Geometry check sheet. Reference: the model listing, model coordinates, mm. A direction names the side the tool comes from. Coordinates: 2 decimals unless noted, no trailing zeros. Order: outer loops, then holes, each group sorted by start corner. A loop starts at its lowest first (then second) coordinate and runs counter-clockwise, first axis right, second up. Notation, with made-up numbers: (0, 18) -> (10, 18) arc R12 cw to (10, 22) -> close; hole circle Ø4 at (-23, 11.25). An arc over 180 degrees is marked (long way). Answer in a Markdown table with one row per item. Add a question column.
```python
from build123d import *

# Parameters (mm, degrees)
F0_R     = 7.5
F1_DEPTH = 10
F2_DEPTH = 20
F3_R     = 2.5
F4_DEPTH = 3.9289322881


with BuildPart() as f1:
    # F0 (on Front) → F1 (new body)
    with BuildSketch(Plane.XZ):
        with BuildLine():
            Line((11.1803398875, 10), (-11.1803398875, 10))
            ThreePointArc((-11.1803398875, 10), (0, -15), (11.1803398875, 10))
        make_face()
        Circle(F0_R, mode=Mode.SUBTRACT)
        with BuildLine():
            ThreePointArc((11.1803398875, 10), (0, -15), (-11.1803398875, 10))
            Line((-11.1803398875, 10), (-20.1556443707, 10))
            ThreePointArc((-20.1556443707, 10), (0, -22.5), (20.1556443707, 10))
            Line((20.1556443707, 10), (11.1803398875, 10))
        make_face()
    extrude(amount=F1_DEPTH)

    # F0 (on Front) → F2 (join)
    with BuildSketch(Plane.XZ):
        with BuildLine():
            Line((11.1803398875, 10), (-11.1803398875, 10))
            ThreePointArc((-11.1803398875, 10), (0, -15), (11.1803398875, 10))
        make_face()
        Circle(F0_R, mode=Mode.SUBTRACT)
    extrude(amount=F2_DEPTH)

    # F3 (on face) → F4 (cut, up to face)
    with BuildSketch(Plane.XY.offset(10)):
        with Locations((0, -15)):
            Circle(F3_R)
    extrude(amount=-F4_DEPTH, mode=Mode.SUBTRACT)


solid = f1.part
```
(1) Cross-section at B-B (x = 0). Enter the section's corners in (y, z).
(2) Go/stop test with flat-tipped pins: P1, Ø8, axis at y = -17.5, z = 0.5, coming from the +X side; P2, Ø1.5, axis at y = -2.5, z = -10, coming from the +X side; P3, Ø4, axis at x = 2.5, z = -11.5, coming from the +Y side; P4, Ø1.5, axis at y = -4, z = -9, coming from the -X side. Record where each tip stops, or that it passes through.
(3) Access from +Z, -Z, +X, -X, +Y, -Y to the whole of each face (thin tool, end or side, straight path). Record for faces 5 (the face through (0, -8, 10)), 6 (the face through (0, -15, -15)).
(4) Cross-section at C-C (y = -8). Enter the section's corners in (x, z).
(5) Scan lines: line 1 along Y through (x, z) = (0, 8); line 2 along Z through (x, y) = (0, -11.5); line 3 along Y through (x, z) = (-12, -16.5). Record each from-to range of solid material in increasing order.
(6) Cross-section at A-A (z = 0). Enter the section's corners in (x, y).
(7) Cross-section at D-D (z = -3.5). Enter the section's corners in (x, y).
(8) Mould release check, pull along X, two halves, no side actions. Record for faces 1 (the face through (0, -10, -17)), 2 (the face through (-0.64, -4.93, -22.49)), 3 (the face through (-0.54, -17.44, 8.56)), 4 (the face through (-1.63, -9.86, -7.32)): +X half, -X half, draft (parallel to the pull), parting line (faces both ways), or undercut.
Checks:
| question | item | result |
|---|---|---|
| 1 | outline | (-20, -15) -> (-10, -15) -> (-10, -22.5) -> (0, -22.5) -> (0, -7.5) -> (-20, -7.5) -> close; (-20, 7.5) -> (-17.5, 7.5) -> (-17.5, 10) -> (-20, 10) -> close; (-12.5, 7.5) -> (0, 7.5) -> (0, 10) -> (-12.5, 10) -> close |
| 2 | P1 | x = 15 |
| 2 | P2 | x = 20.51 |
| 2 | P3 | y = 0 |
| 2 | P4 | x = -20.93 |
| 3 | face 5 | +Z, +X, -X, +Y, -Y |
| 3 | face 6 | -Y |
| 4 | outline | (-20.16, 10) arc R22.5 ccw (long way) to (20.16, 10) -> close; hole circle Ø15 at (0, 0) |
| 5 | line 1 | -20 to -17.5, -12.5 to 0 |
| 5 | line 2 | -15 to -7.5, 7.5 to 10 |
| 5 | line 3 | -10 to 0 |
| 6 | outline | (-22.5, -10) -> (-15, -10) -> (-15, -20) -> (-7.5, -20) -> (-7.5, 0) -> (-22.5, 0) -> close; (7.5, -20) -> (15, -20) -> (15, -10) -> (22.5, -10) -> (22.5, 0) -> (7.5, 0) -> close |
| 7 | outline | (-22.23, -10) -> (-14.59, -10) -> (-14.59, -20) -> (-6.63, -20) -> (-6.63, 0) -> (-22.23, 0) -> close; (6.63, -20) -> (14.59, -20) -> (14.59, -10) -> (22.23, -10) -> (22.23, 0) -> (6.63, 0) -> close |
| 8 | face 1 | draft |
| 8 | face 2 | parting line |
| 8 | face 3 | undercut |
| 8 | face 4 | undercut |
